For this review, take the finished solid that the model builds, in its own axes (mm). Face numbers are marked on the shaded views. A direction names the side the tool comes from. Coordinates: 2 decimals unless noted, no trailing zeros. Order: outer loops, then holes, each group sorted by start corner. A loop starts at its lowest first (then second) coordinate and runs counter-clockwise, first axis right, second up. Notation, with made-up numbers: (-30, 84) -> (-6, 84) arc R23 cw to (-6, 123) -> close; hole circle Ø3 at (9.5, 11.25). An arc over 180 degrees is marked (long way). Return JSON: item names as keys, results as strings. Group by question number.
Item 1: Take a section at A-A (x = -11). Write out the cut boundary in (y, z).
Item 2: Draft analysis for pull direction X (two halves, no side actions). For the marked faces 3, 4 and 5, state which applies: +X half, -X half, draft (parallel to the pull), parting line (faces both ways), or undercut.
Item 3: Machinability: for the marked faces 1 and 2, which of the approach directions +Z, -Z, +X, -X, +Y, -Y give a long, thin tool a straight path to every point of the face, cutting with its end or side? Answer none if there is none.
Item 4: Take a section at D-D (y = 13.75). Write out the cut boundary in (x, z), then the cut area to 3 significant figures.
Item 5: Take a section at B-B (y = 5.25). Write out the cut boundary in (x, z), then the cut area to 3 significant figures.
Item 6: Take a section at C-C (z = -6). Write out the cut boundary in (x, y).
Item 7: For line 1 along Z through (x, y) = (-13, 15.5); line 2 along X through (y, z) = (15, -9); line 3 along Z through (x, y) = (17.5, 13.5), list the stretches that pass through material, from the lowest coordinate up.
```python
from build123d import *

# Parameters (mm, degrees)
IZIM1_W                     = 45
IZIM1_H                     = 60
Y_KSEKLIK_EKSTR_ZYON1_DEPTH = 2
IZIM2_W                     = 45
IZIM2_H                     = 60
IZIM2_W_2                   = 42.48
IZIM2_H_2                   = 56.64
Y_KSEKLIK_EKSTR_ZYON2_DEPTH = 18
IZIM6_W                     = 11.5
IZIM6_H                     = 9.5
KES_EKSTR_ZYON2_DEPTH       = 18
IZIM7_W                     = 11
IZIM7_H                     = 3
Y_KSEKLIK_EKSTR_ZYON3_DEPTH = 18


with BuildPart() as part:
    # Çizim1 → Yükseklik-Ekstrüzyon1 (new body)
    with BuildSketch(Plane(origin=(0, 0, 0), x_dir=(1, 0, 0), z_dir=(0, 1, 0))):
        Rectangle(IZIM1_W, IZIM1_H)
    extrude(amount=Y_KSEKLIK_EKSTR_ZYON1_DEPTH)

    # Çizim2 → Yükseklik-Ekstrüzyon2 (add)
    with BuildSketch(Plane(origin=(0, 2, 0), x_dir=(1, 0, 0), z_dir=(0, 1, 0))):
        Rectangle(IZIM2_W, IZIM2_H)
        Rectangle(IZIM2_W_2, IZIM2_H_2, mode=Mode.SUBTRACT)
    extrude(amount=Y_KSEKLIK_EKSTR_ZYON2_DEPTH)

    # Çizim6 → Kes-Ekstrüzyon2 (cut)
    with BuildSketch(Plane.XY.offset(30)):
        with Locations((-15.49, 6.75)):
            Rectangle(IZIM6_W, IZIM6_H)
    extrude(amount=-KES_EKSTR_ZYON2_DEPTH, mode=Mode.SUBTRACT)

    # Çizim7 → Yükseklik-Ekstrüzyon3 (add)
    with BuildSketch(Plane(origin=(0, 2, 0), x_dir=(1, 0, 0), z_dir=(0, 1, 0))):
        with Locations((-15.74, -11.82)):
            Rectangle(IZIM7_W, IZIM7_H)
    extrude(amount=Y_KSEKLIK_EKSTR_ZYON3_DEPTH)


solid = part.part
```
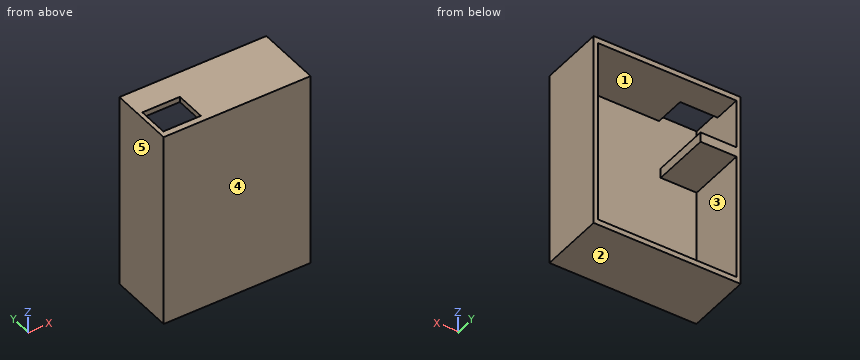
Findings below:
{
 "1": {"outline": "(0, -30) -> (20, -30) -> (20, -28.32) -> (2, -28.32) -> (2, 10.32) -> (20, 10.32) -> (20, 13.32) -> (2, 13.32) -> (2, 30) -> (0, 30) -> close; (11.5, 28.32) -> (20, 28.32) -> (20, 30) -> (11.5, 30) -> close"},
 "2": {"face 3": "undercut", "face 4": "draft", "face 5": "-X half"},
 "3": {"face 1": "+Y", "face 2": "-Z, +X, -X, +Y, -Y"},
 "4": {"outline": "(-22.5, -30) -> (22.5, -30) -> (22.5, 30) -> (-22.5, 30) -> close; hole (-21.24, -28.32) -> (21.24, -28.32) -> (21.24, 28.32) -> (-21.24, 28.32) -> (-21.24, 13.32) -> (-10.24, 13.32) -> (-10.24, 10.32) -> (-21.24, 10.32) -> close", "area": "327 mm2"},
 "5": {"outline": "(-22.5, -30) -> (22.5, -30) -> (22.5, 30) -> (-9.74, 30) -> (-9.74, 28.32) -> (21.24, 28.32) -> (21.24, -28.32) -> (-21.24, -28.32) -> (-21.24, 10.32) -> (-10.24, 10.32) -> (-10.24, 13.32) -> (-21.24, 13.32) -> (-21.24, 30) -> (-22.5, 30) -> close", "area": "308 mm2"},
 "6": {"outline": "(-22.5, 0) -> (22.5, 0) -> (22.5, 20) -> (21.24, 20) -> (21.24, 2) -> (-21.24, 2) -> (-21.24, 20) -> (-22.5, 20) -> close"},
 "7": {"line 1": "z = -30 to -28.32, 10.32 to 13.32, 28.32 to 30", "line 2": "x = -22.5 to -21.24, 21.24 to 22.5", "line 3": "z = -30 to -28.32, 28.32 to 30"}
}
